```python
from build123d import *

# Parameters (mm, degrees)
F1_DEPTH  = 25.4
F3_DEPTH  = 25.4
F5_DEPTH  = 25.4
F7_DEPTH  = 25.4
F9_DEPTH  = 50.8
F11_DEPTH = 27.178
F13_DEPTH = 25.4
F14_R     = 6.1753595884
F15_DEPTH = 50.8


with BuildPart() as f1:
    # F0 (on Front) → F1 (new body)
    with BuildSketch(Plane.XZ):
        Polygon((-42.333334913, 38.1), (-42.333334913, 0), (46.566665087, 0), (46.566665087, 11.0066671406), (-16.933334913, 11.0066671406), (-16.933334913, 38.1), align=None)
    extrude(amount=F1_DEPTH)

    # F2 (on face) → F3 (cut)
    with BuildSketch(Plane.XZ.offset(25.4)):
        with BuildLine():
            ThreePointArc((-37.9148391216, 0), (-40.8140278818, 1.5211007742), (-42.333334913, 4.4212299399))
            Line((-42.333334913, 4.4212299399), (-42.333334913, 0))
            Line((-42.333334913, 0), (-37.9148391216, 0))
        make_face()
    extrude(amount=-F3_DEPTH, mode=Mode.SUBTRACT)

    # F4 (on face) → F5 (cut)
    with BuildSketch(Plane.XY.offset(11.0066671406)):
        with BuildLine():
            ThreePointArc((34.7993597388, 0), (45.3010079388, -11.6808324), (37.6517660916, -25.4))
            Line((37.6517660916, -25.4), (46.566665087, -25.4))
            Line((46.566665087, -25.4), (46.566665087, 0))
            Line((46.566665087, 0), (34.7993597388, 0))
        make_face()
    extrude(amount=-F5_DEPTH, mode=Mode.SUBTRACT)

    # F6 (on face) → F7 (cut)
    with BuildSketch(Plane.XY.offset(38.1)):
        with BuildLine():
            ThreePointArc((-16.933334913, -24.7742129951), (-12.9263389557, -18.5421251923), (-11.5236387204, -11.2670054659))
            ThreePointArc((-11.5236387204, -11.2670054659), (-49.0871210436, -3.583342718), (-17.5579703651, -25.4))
            Line((-17.5579703651, -25.4), (-42.333334913, -25.4))
            Line((-42.333334913, -25.4), (-42.333334913, 0))
            Line((-42.333334913, 0), (-16.933334913, 0))
            Line((-16.933334913, 0), (-16.933334913, -24.7742129951))
        make_face()
    extrude(amount=-F7_DEPTH, mode=Mode.SUBTRACT)

    # F8 (on face) → F9 (cut)
    with BuildSketch(Plane.XY.offset(38.1)):
        with BuildLine():
            ThreePointArc((-42.333334913, -11.1485840045), (-39.2676835177, -4.1212770864), (-32.8026749194, 0))
            Line((-32.8026749194, 0), (-42.333334913, 0))
            Line((-42.333334913, 0), (-42.333334913, -11.1485840045))
        make_face()
        with BuildLine():
            ThreePointArc((-32.5174331665, -25.4), (-39.1711473149, -21.3143901639), (-42.333334913, -14.1754344072))
            Line((-42.333334913, -14.1754344072), (-42.333334913, -25.4))
            Line((-42.333334913, -25.4), (-32.5174331665, -25.4))
        make_face()
    extrude(amount=-F9_DEPTH, mode=Mode.SUBTRACT)

    # F10 (on face) → F11 (cut)
    with BuildSketch(Plane.XY.offset(38.1)):
        with BuildLine():
            ThreePointArc((-24.8680049162, 0), (-19.4963079038, -4.4575302948), (-16.933334913, -10.95028584))
            Line((-16.933334913, -10.95028584), (-16.933334913, 0))
            Line((-16.933334913, 0), (-24.8680049162, 0))
        make_face()
        with BuildLine():
            ThreePointArc((-16.933334913, -14.44971416), (-19.4963079038, -20.9424697052), (-24.8680049162, -25.4))
            Line((-24.8680049162, -25.4), (-16.933334913, -25.4))
            Line((-16.933334913, -25.4), (-16.933334913, -14.44971416))
        make_face()
    extrude(amount=-F11_DEPTH, mode=Mode.SUBTRACT)

    # F12 (on face) → F13 (cut)
    with BuildSketch(Plane.XY.offset(11.0066671406)):
        with BuildLine():
            ThreePointArc((0, 2.0500258297), (-2.7772999757, 1.5187665416), (-5.1624582049, 0))
            Line((-5.1624582049, 0), (5.1624582049, 0))
            ThreePointArc((5.1624582049, 0), (2.7772999757, 1.5187665416), (0, 2.0500258297))
        make_face()
        with BuildLine():
            ThreePointArc((0, 2.0500258297), (2.7772999757, 1.5187665416), (5.1624582049, 0))
            Line((5.1624582049, 0), (15.1562278536, 0))
            ThreePointArc((15.1562278536, 0), (17.6040380518, 1.6191667448), (20.4805661222, 2.2014570285))
            Line((20.4805661222, 2.2014570285), (0, 2.0500258297))
        make_face()
        with BuildLine():
            ThreePointArc((20.4805661222, 2.2014570285), (17.6040380518, 1.6191667448), (15.1562278536, 0))
            Line((15.1562278536, 0), (25.9184243712, 0))
            ThreePointArc((25.9184243712, 0), (23.4180808332, 1.6406606681), (20.4805661222, 2.2014570285))
        make_face()
    extrude(amount=-F13_DEPTH, mode=Mode.SUBTRACT)

    # F14 (on face) → F15 (cut)
    with BuildSketch(Plane.XY.offset(38.1)):
        with Locations((-29.2770774571, -12.6620092059)):
            Circle(F14_R)
    extrude(amount=-F15_DEPTH, mode=Mode.SUBTRACT)


solid = f1.part
```
Could you check a few things on this model? Use its own coordinates, in mm. A direction names the side the tool comes from. Coordinates: 2 decimals unless noted, no trailing zeros. Write each loop counter-clockwise with the first axis right and the second up, starting at its lowest first coordinate (ties: lowest second). Pieces come first, ordered by that corner, then holes. Notation, with made-up numbers: (-10.75, -32) - (11.25, -32) arc R22 ccw to (11.25, -10) - close; hole circle Ø5 at (-34, 52). An arc over 180 degrees is marked (long way). Use a Markdown table: item, result.
Q1. Which directions (+Z, -Z, +X, -X, +Y, -Y) give clear straight access to the entire face, cutting with the end or side of a thin tool? Please do faces 5 (the flat face through (-6.99, 0, 10.85)), 6 (the flat face through (-16.933, -13, 24)), 7 (the flat face through (-19, -3, 10.922)).
Geometry check:
| item | result |
|---|---|
| face 5 | +Z, -Z, +X, -X, +Y |
| face 6 | +Z, +X, +Y, -Y |
| face 7 | +Z, +Y |
Q2. Thinking about a two-plate mould opening in X: for faces 1 (the flat face through (-19, -22, 10.922)), 2 (the cylindrical face through (-40.221, -12.801, 1.007)), 3 (the cylindrical face through (-23.387, -10.807, 19.317)), 4 (the flat face through (15, -13, 11.007)), which applies, +X half, -X half, draft (parallel to the pull), parting line (faces both ways), or undercut?
Geometry check:
| item | result |
|---|---|
| face 1 | undercut |
| face 2 | -X half |
| face 3 | undercut |
| face 4 | draft |
Q3. Imagine slicing it at D-D (x = 27.5). List the corners of the cut face in (y, z) for me, and give its area (3 significant figures).
Geometry check:
| item | result |
|---|---|
| outline | (-25.4, 0) - (0, 0) - (0, 11.01) - (-25.4, 11.01) - close |
| area | 280 mm2 |
Q4. Imagine slicing it at B-B (z = 13). List the corners of the cut face in (x, y) for me.
Geometry check:
| item | result |
|---|---|
| outline | (-42.33, -14.18) arc R13.14 ccw to (-32.52, -25.4) - (-24.87, -25.4) arc R14.05 ccw to (-16.93, -14.45) - (-16.93, -10.95) arc R14.05 ccw to (-24.87, 0) - (-32.8, 0) arc R13.14 ccw to (-42.33, -11.15) - close; hole circle Ø12.35 at (-29.28, -12.66) |
Q5. Imagine slicing it at C-C (y = -19.75). List the corners of the cut face in (x, z) for me.
Geometry check:
| item | result |
|---|---|
| outline | (-40.35, 1.1) arc R5.49 ccw to (-37.91, 0) - (43.68, 0) - (43.68, 11.01) - (-16.93, 11.01) - (-16.93, 10.92) - (-18.72, 10.92) - (-18.72, 38.1) - (-40.35, 38.1) - close |
Q6. Please list where these lines run through material, in increasing order: L1, parallel to Z at x = -2.5, y = -4; L2, parallel to Y at x = -33, z = 34; L3, parallel to Y at x = -30.5, z = 31.
Geometry check:
| item | result |
|---|---|
| L1 | z = 0 to 11.01 |
| L2 | y = -25.27 to -17.59, -7.74 to -0.06 |
| L3 | y = -25.4 to -18.72, -6.61 to 0 |
Q7. I'm going to push flat-ended pins straight in: pin 1 Ø4 at (y, z) = (-20.5, 26) entering from +X; pin 2 Ø4 at (x, y) = (-19.5, -21.5) entering from +Z; pin 3 Ø1.7 at (y, z) = (-13, 22) entering from +X; pin 4 Ø5 at (y, z) = (-18.5, 22.5) entering from +X. Where does each tip first touch, or does it pass through?
Geometry check:
| item | result |
|---|---|
| pin 1 | stops at x = -18.08 |
| pin 2 | stops at z = 38.1 |
| pin 3 | stops at x = -16.93 |
| pin 4 | stops at x = -17.22 |
Q8. Imagine slicing it at A-A (x = -31). List the corners of the cut face in (y, z) for me, and give its area (3 significant figures).
Geometry check:
| item | result |
|---|---|
| outline | (-25.4, 0) - (-18.59, 0) - (-18.59, 38.1) - (-25.4, 38.1) - close; (-6.73, 0) - (0, 0) - (0, 38.1) - (-6.73, 38.1) - close |
| area | 516 mm2 |
